Build history of the part. All positions in model axes, mm. A direction names the side the tool comes from. Give positions to 0.01 mm unless a question says otherwise; leave off trailing zeros. Write each loop counter-clockwise with the first axis right and the second up, starting at its lowest first coordinate (ties: lowest second). Pieces come first, ordered by that corner, then holes. Notation, with made-up numbers: M 54,33 L 73,33 A16 cw 73,53 Z; hole C 3.5,82.5 d6. An arc over 180 degrees is marked long. Return JSON: item names as keys, results as strings. Group by question number.
Q1. Band-saw the part on A-A, the plane x = 2.5. Give the cut face in (y, z).
Q2. Pull direction Y, two halves, no side cores. Call faces 1 (the flat face through (5, 2.2, 2.5)), 2 (the cylindrical face through (0.07, 5.96, 3.67)), 3 (the cylindrical face through (-0.063, 10.492, -3.304)): +Y half, -Y half, draft (parallel to the pull), parting line (faces both ways), or undercut.
Q3. Flat gauge pins, fed straight in: pin 1 Ø2 at (x, z) = (2, -4.5) entering from +Y; pin 2 Ø6 at (x, y) = (0, -5.5) entering from +Z; pin 3 Ø1 at (y, z) = (-1.5, -1.5) entering from +X. Where does each tip first touch, or does it go through?
Q4. Band-saw the part on B-B, the plane z = 0. Count the separate pieces of the cut face and the enclosed holes in it, then the cut area to 3 significant figures.
Q5. Wall check: probe 1 along Y at (x, z) = (-0.25, 0.75); probe 2 along Z at (x, y) = (-0.5, 4.25); probe 3 along Z at (x, y) = (-1.5, -1). Give the ranges that are in metal, low to high.
Q6. Tool access for faces 4 (the cylindrical face through (0.066, -6.327, 0.369)), 5 (the cylindrical face through (0.04, 2.91, 0.08)): list every direction of +Z, -Z, +X, -X, +Y, -Y with a clear straight run to the whole face (end or side of a thin tool).
Autodesk Inventor part; units mm, degrees
ref_plane "body_set_h_XY" through (0, -7.7782, 7.7782) normal (0, 0.7071, -0.7071) x (1, 0, 0)
ref_plane "body_set_h_YZ" through (0, -7.7782, 7.7782) normal (1, 0, 0) x (0, -0.7071, -0.7071)
ref_plane "body_set_h_ZX" through (0, -7.7782, 7.7782) normal (0, -0.7071, -0.7071) x (0, 0.7071, -0.7071)
sketch "Sketch_1" plane through (0, 0, 0) normal (0, 0, 1) x (1, 0, 0)
  line L0 (0, 0) -> (-5, 0)
  line L1 (-5, 3) -> (-4.5, 2.5)
  line L2 (-4.5, 2.5) -> (4.5, 2.5)
  line L3 (4.5, 2.5) -> (5, 3)
  line L4 (5, 3) -> (5, 10.5)
  line L5 (5, 10.5) -> (4.5, 11)
  line L6 (4.5, 11) -> (-4.5, 11)
  line L7 (-4.5, 11) -> (-5, 10.5)
  line L8 (-5, 10.5) -> (-5, 3)
revolve "Revolution1" add sketch "Sketch_1" angle 360 about axis through (0, 0, 0) along (1, 0, 0)
sketch "Sketch_2" plane through (0, 0, 0) normal (1, 0, 0) x (0, 1, 0)
  line L0 (8.556, 8.556) -> (0.9899, 0.9899)
  line L1 (0.9899, 0.9899) -> (-0.4243, 2.4042)
  line L2 (-0.4243, 2.4042) -> (0.3536, 3.182)
  line L3 (0.3536, 3.182) -> (0.8895, 3.182)
  line L4 (0.8895, 3.182) -> (6.364, 8.6564)
  line L5 (6.364, 8.6564) -> (6.364, 9.1924)
  line L6 (6.364, 9.1924) -> (7.1418, 9.9702)
  line L7 (7.1418, 9.9702) -> (8.556, 8.556)
  line L8 (8.556, 8.556) -> (0.9899, 0.9899)
revolve "Revolution2" cut sketch "Sketch_2" angle 360 about axis through (0, 8.556, 8.556) along (0, 0.7071, 0.7071)
thread "Thread1"
sketch "Sketch_3" plane through (0, 0, 0) normal (1, 0, 0) x (0, 1, 0)
  line L0 (-8.556, 8.556) -> (-0.9899, 0.9899)
  line L1 (-0.9899, 0.9899) -> (-2.4042, -0.4243)
  line L2 (-2.4042, -0.4243) -> (-3.182, 0.3536)
  line L3 (-3.182, 0.3536) -> (-3.182, 0.8895)
  line L4 (-3.182, 0.8895) -> (-8.6564, 6.364)
  line L5 (-8.6564, 6.364) -> (-9.1924, 6.364)
  line L6 (-9.1924, 6.364) -> (-9.9702, 7.1418)
  line L7 (-9.9702, 7.1418) -> (-8.556, 8.556)
  line L8 (-8.556, 8.556) -> (-0.9899, 0.9899)
revolve "Revolution3" cut sketch "Sketch_3" angle 360 about axis through (0, -8.556, 8.556) along (0, -0.7071, 0.7071)
thread "Thread2"
sketch "Sketch_10" plane through (0, 0, 0) normal (0, 1, 0) x (-1, 0, 0)
  line L0 (-5, -7.5) -> (5, -7.5)
  line L1 (5, -7.5) -> (5, -9)
  line L2 (5, -9) -> (4.7295, -8.7295)
  line L3 (4.7295, -8.7295) -> (-4.7295, -8.7295)
  line L4 (-4.7295, -8.7295) -> (-5, -9)
  line L5 (-5, -9) -> (-5, -7.5)
  line L6 (-5, -7.5) -> (5, -7.5)
revolve "Revolution4" cut sketch "Sketch_10" angle 360 about axis through (5, 0, -7.5) along (1, 0, 0)
thread "Thread3"
sketch "Sketch_11" plane through (0, 0, 0) normal (0, 1, 0) x (-1, 0, 0)
  line L0 (-5, 7.5) -> (5, 7.5)
  line L1 (5, 7.5) -> (5, 6)
  line L2 (5, 6) -> (4.7295, 6.2705)
  line L3 (4.7295, 6.2705) -> (-4.7295, 6.2705)
  line L4 (-4.7295, 6.2705) -> (-5, 6)
  line L5 (-5, 6) -> (-5, 7.5)
  line L6 (-5, 7.5) -> (5, 7.5)
revolve "Revolution5" cut sketch "Sketch_11" angle 360 about axis through (5, 0, 7.5) along (1, 0, 0)
thread "Thread4"
sketch "Sketch_12" plane through (0, 0, 0) normal (0, 0, 1) x (1, 0, 0)
  line L0 (5, 7.5) -> (-5, 7.5)
  line L1 (-5, 7.5) -> (-5, 9)
  line L2 (-5, 9) -> (-4.7295, 8.7295)
  line L3 (-4.7295, 8.7295) -> (4.7295, 8.7295)
  line L4 (4.7295, 8.7295) -> (5, 9)
  line L5 (5, 9) -> (5, 7.5)
  line L6 (5, 7.5) -> (-5, 7.5)
revolve "Revolution6" cut sketch "Sketch_12" angle 360 about axis through (5, 7.5, 0) along (1, 0, 0)
thread "Thread5"
sketch "Sketch_13" plane through (0, 0, 0) normal (0, 0, 1) x (1, 0, 0)
  line L0 (5, -7.5) -> (-5, -7.5)
  line L1 (-5, -7.5) -> (-5, -6)
  line L2 (-5, -6) -> (-4.7295, -6.2705)
  line L3 (-4.7295, -6.2705) -> (4.7295, -6.2705)
  line L4 (4.7295, -6.2705) -> (5, -6)
  line L5 (5, -6) -> (5, -7.5)
  line L6 (5, -7.5) -> (-5, -7.5)
revolve "Revolution7" cut sketch "Sketch_13" angle 360 about axis through (5, -7.5, 0) along (1, 0, 0)
thread "Thread6"
ref_plane "body_set_h_XY" through (0, -7.7782, 7.7782) normal (0, 0.7071, -0.7071) x (1, 0, 0)
ref_plane "body_set_h_YZ" through (0, -7.7782, 7.7782) normal (1, 0, 0) x (0, -0.7071, -0.7071)
ref_plane "body_set_h_ZX" through (0, -7.7782, 7.7782) normal (0, -0.7071, -0.7071) x (0, 0.7071, -0.7071)
ref_plane "body_set_v_XY" through (0, 7.7782, 7.7782) normal (0, 0.7071, 0.7071) x (1, 0, 0)
ref_plane "body_set_v_YZ" through (0, 7.7782, 7.7782) normal (1, 0, 0) x (0, 0.7071, -0.7071)
ref_plane "body_set_v_ZX" through (0, 7.7782, 7.7782) normal (0, 0.7071, -0.7071) x (0, 0.7071, 0.7071)
properties part number "SCMW5b"
From the geometry:
{
 "1": {"outline": "C 0,0 d22; hole C -7.5,0 d2.46; hole C 0,0 d5; hole C 0,-7.5 d2.46; hole C 0,7.5 d2.46; hole C 7.5,0 d2.46"},
 "2": {"face 1": "draft", "face 2": "undercut", "face 3": "parting line"},
 "3": {"pin 1": "stops at y = 10.43", "pin 2": "stops at z = 10.71", "pin 3": "stops at x = 4.62"},
 "4": {"separate pieces": "4", "enclosed holes": "0", "area": "119 mm^2"},
 "5": {"probe 1": "y = -10.97 to -8.47, -6.53 to -3.17, 3.17 to 6.53, 8.47 to 10.97", "probe 2": "z = -10.15 to 2.07, 6.43 to 10.15", "probe 3": "z = -10.95 to -8.22, -6.78 to -2.29, 2.67 to 6.78, 8.22 to 10.95"},
 "6": {"face 4": "+X, -X", "face 5": "none"}
}
